Design review of the part built by this model. Coordinates are the model's own, in mm. A direction names the side the tool comes from. Coordinates: 2 decimals unless noted, no trailing zeros. Write each loop counter-clockwise with the first axis right and the second up, starting at its lowest first coordinate (ties: lowest second). Pieces come first, ordered by that corner, then holes.
Q1. For probe 1 along Y at (x, z) = (0, 41); probe 2 along X at (y, z) = (0, 6); probe 3 along X at (y, z) = (0, 10), list the stretches that pass through material, from the lowest coordinate up.
Q2. Take a section at C-C (z = 16). Give the boundary of the cut face in (x, y) (1 decimal).
Q3. Insertion check: pin 1 (1 mm diameter, centred on x = 0.5, y = -0.5, fed in from -Z) (3 decimals); pin 2 (6 mm diameter, centred on x = -23, y = 17.5, fed in from -Z); pin 3 (3 mm diameter, centred on x = 2, y = 1, fed in from +Z) (3 decimals). Each pin has a flat end and moves straight along its axis. Give the tip position at first contact, or say it passes through.
Q4. Machinability: for faces 1 (the cylindrical face through (-9.84, 7.54, 41.5)), 2 (the cylindrical face through (-0.34, -1.55, 11.91)), 3 (the flat face through (0, 5, 45.72)), which of the approach directions +Z, -Z, +X, -X, +Y, -Y give a long, thin tool a straight path to every point of the face, cutting with its end or side? Answer none if there is none.
Q5. Mouldability with a two-part tool opening along X and no side actions: class faces 4 (the flat face through (0, 0, 22.225)), 5 (the cylindrical face through (-6.883, 30.995, 32.15)), 6 (the flat face through (14, 0, 37.159)) as pulls with the +X half, pulls with the -X half, needs draft (parallel to the pull), parting line crosses it, or undercut.
```python
from build123d import *

# Parameters (mm, degrees)
F2_R     = 4.7625
F3_DEPTH = 9.525
F4_R     = 1.5875
F5_DEPTH = 22.225


with BuildPart() as f1:
    # F0 (on Front) → F1 (revolve)
    with BuildSketch(Plane.XZ):
        Polygon((0, 45.72), (0, 0), (5.08, 6.010141), (12.395916, 19.379321), (31.75, 26.999321), (31.75, 37.159321), (12.395916, 37.159321), (12.395916, 45.72), align=None)
    revolve(axis=Axis((0, 0, 22.86), (0, 0, -1)))

    # F2 (on face) → F3 (cut)
    with BuildSketch(Plane.XY.offset(45.72)):
        Circle(F2_R)
    extrude(amount=-F3_DEPTH, mode=Mode.SUBTRACT)

    # F4 (on Top) → F5 (cut)
    with BuildSketch(Plane.XY):
        Circle(F4_R)
    extrude(amount=F5_DEPTH, mode=Mode.SUBTRACT)


solid = f1.part
```
Response:
1. probe 1: y = -12.4 to -4.76, 4.76 to 12.4
1. probe 2: x = -5.07 to -1.59, 1.59 to 5.07
1. probe 3: x = -7.26 to -1.59, 1.59 to 7.26
2. outline: circle Ø21.1 at (0, 0); hole circle Ø3.2 at (0, 0)
3. pin 1: stops at z = 22.225
3. pin 2: stops at z = 24.7
3. pin 3: stops at z = 36.195
4. face 1: +Z
4. face 2: -Z
4. face 3: +Z, +X, -X, +Y, -Y
5. face 4: undercut
5. face 5: parting line crosses it
5. face 6: needs draft
